Read the model definition and answer for the solid it produces. Units are mm, in the model's axes. Face numbers are marked on the shaded views. A direction names the side the tool comes from. Coordinates: 2 decimals unless noted, no trailing zeros. Write each loop counter-clockwise with the first axis right and the second up, starting at its lowest first coordinate (ties: lowest second). Pieces come first, ordered by that corner, then holes. Notation, with made-up numbers: M 40,47 L 97,47 A8 ccw 97,57 Z; hole C 25,11 d6. An arc over 180 degrees is marked long. Use a Markdown table: item, result. Add a question column.
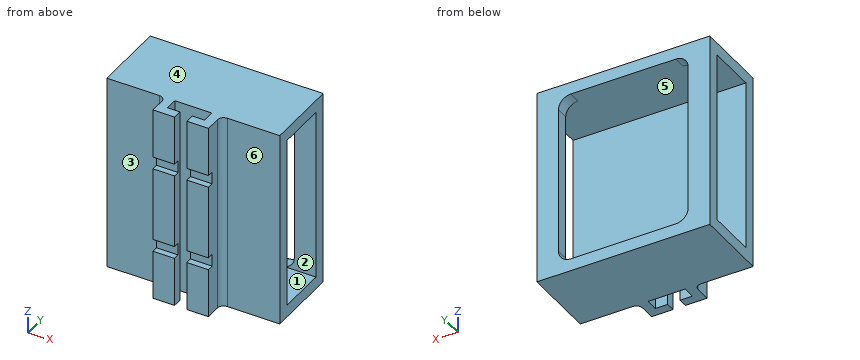
from build123d import *

# Parameters (mm, degrees)
SKETCH_1_W          = 28
SKETCH_1_H          = 12
SKETCH_1_W_2        = 9
SKETCH_1_H_2        = 3.5
EXTRUDE_1_DEPTH     = 32
SKETCH_2_W          = 1
SKETCH_2_H          = 1.5
CUT_EXTRUDE_1_DEPTH = 37.197375595
SKETCH_3_W          = 2
SKETCH_3_H          = 1
CUT_EXTRUDE_2_DEPTH = 39.164119275
FILLET_1_R          = 1
SKETCH_6_W          = 28
SKETCH_6_H          = 8
CUT_EXTRUDE_5_DEPTH = 44.568910934
CUT_EXTRUDE_4_REACH = 40.213
SKETCH_5_W          = 21
SKETCH_5_H          = 28
FILLET_2_R          = 2


with BuildPart() as part:
    # 草图1 → 凸台-拉伸1 (new body)
    with BuildSketch(Plane.XY):
        Rectangle(SKETCH_1_W, SKETCH_1_H)
        with Locations((0, -7.75)):
            Rectangle(SKETCH_1_W_2, SKETCH_1_H_2)
    extrude(amount=EXTRUDE_1_DEPTH)

    # 草图2 → 切除-拉伸1 (cut, through all)
    with BuildSketch(Plane(origin=(0, 0, 0), x_dir=(-1, 0, 0), z_dir=(0, 0, -1))):
        Polygon((0, -6), (-3, -6), (-3, -8), (-1, -8), (0, -8), align=None)
        Polygon((3, -6), (0, -6), (0, -8), (1, -8), (3, -8), align=None)
        with Locations((-0.5, -8.75)):
            Rectangle(SKETCH_2_W, SKETCH_2_H)
        with Locations((0.5, -8.75)):
            Rectangle(SKETCH_2_W, SKETCH_2_H)
    extrude(amount=-CUT_EXTRUDE_1_DEPTH, mode=Mode.SUBTRACT)

    # 草图3 → 切除-拉伸2 (cut, through all)
    with BuildSketch(Plane.ZY.offset(4.5)):
        with Locations((9, -9)):
            Rectangle(SKETCH_3_W, SKETCH_3_H)
        with Locations((23, -9)):
            Rectangle(SKETCH_3_W, SKETCH_3_H)
    extrude(amount=-CUT_EXTRUDE_2_DEPTH, mode=Mode.SUBTRACT)

    # 圆角1
    fillet_1_edges = [part.edges().sort_by_distance(p)[0] for p in [
        (4.5, -6, 16),
        (-4.5, -6, 16),
    ]]
    fillet(fillet_1_edges, radius=FILLET_1_R)

    # 草图6 → 切除-拉伸5 (cut, through all)
    with BuildSketch(Plane(origin=(14, 0, 0), x_dir=(0, 0, -1), z_dir=(1, 0, 0))):
        with Locations((-16, 0)):
            Rectangle(SKETCH_6_W, SKETCH_6_H)
    extrude(amount=-CUT_EXTRUDE_5_DEPTH, mode=Mode.SUBTRACT)

    # 草图5 → 切除-拉伸4 (cut, up to next)
    with BuildSketch(Plane(origin=(0, 6, 0), x_dir=(1, 0, 0), z_dir=(0, 1, 0)), mode=Mode.PRIVATE) as cut_extrude_4_sk1:
        with Locations((0, -16)):
            Rectangle(SKETCH_5_W, SKETCH_5_H)
    cut_extrude_4_tool1 = extrude(cut_extrude_4_sk1.sketch, amount=-CUT_EXTRUDE_4_REACH, mode=Mode.PRIVATE) & part.part
    add(cut_extrude_4_tool1.solids().sort_by_distance((0, 6, 16))[0], mode=Mode.SUBTRACT)

    # 圆角2
    fillet_2_edges = [part.edges().sort_by_distance(p)[0] for p in [
        (10.5, 5, 30),
        (10.5, 5, 2),
        (-10.5, 5, 2),
        (-10.5, 5, 30),
    ]]
    fillet(fillet_2_edges, radius=FILLET_2_R)


solid = part.part
Item 1: Find section B-B on z = 15. Give the vertices of the cut face in (x, y), then the cut area to 3 significant figures.
Item 2: Find section C-C on x = -2.25. Give the vertices of the cut face in (y, z), then the cut area to 3 significant figures.
Item 3: Each of these flat-tipped pins is pushed along its axis until it touches: pin 1 (4 mm diameter, centred on x = 12, z = 8, fed in from -Y); pin 2 (2 mm diameter, centred on y = -7.5, z = 10, fed in from +X); pin 3 (1.5 mm diameter, centred on x = 1, z = 11, fed in from +Y); pin 4 (0.8 mm diameter, centred on x = -3, y = -9, fed in from -Z). Where does it stop, or does it pass through?
Item 4: Consider probe 1 along Z at (x, y) = (9, 3.25); probe 2 along Y at (x, z) = (11, 28); probe 3 along Y at (x, z) = (-10, 14.5). Determine where each line is inside the solid, lowest interval first.
Item 5: Find section A-A on y = 2.75. Give the vertices of the cut face in (x, z), then the cut area to 3 significant figures.
Item 6: Determine the mould class of the marked faces 4, 5 and 6 for opening direction Z: pulls with the +Z half, pulls with the -Z half, needs draft (parallel to the pull), parting line crosses it, or undercut.
Item 7: For the marked faces 1, 2 and 3, determine the directions among +Z, -Z, +X, -X, +Y, -Y from which every point of the face is accessible in a straight line to the end or side of a thin tool.
Item 8: Find section D-D on x = 6.5. Give the vertices of the cut face in (y, z).
Geometry says:
| question | item | result |
|---|---|---|
| 1 | outline | M -14,-6 L -5.5,-6 A1 cw -4.5,-7 L -4.5,-9.5 L -1,-9.5 L -1,-8 L -3,-8 L -3,-6 L 3,-6 L 3,-8 L 1,-8 L 1,-9.5 L 4.5,-9.5 L 4.5,-7 A1 cw 5.5,-6 L 14,-6 L 14,-4 L -14,-4 Z; M -14,4 L -10.5,4 L -10.5,6 L -14,6 Z; M 10.5,4 L 14,4 L 14,6 L 10.5,6 Z |
| 1 | area | 86.9 mm2 |
| 2 | outline | M -9.5,0 L -8,0 L -8,32 L -9.5,32 L -9.5,24 L -8.5,24 L -8.5,22 L -9.5,22 L -9.5,10 L -8.5,10 L -8.5,8 L -9.5,8 Z; M -6,0 L 6,0 L 6,2 L -4,2 L -4,30 L 6,30 L 6,32 L -6,32 Z |
| 2 | area | 148 mm2 |
| 3 | pin 1 | stops at y = -6 |
| 3 | pin 2 | stops at x = 4.63 |
| 3 | pin 3 | stops at y = -4 |
| 3 | pin 4 | stops at z = 0 |
| 4 | probe 1 | z = 0 to 2, 30 to 32 |
| 4 | probe 2 | y = -6 to -4, 4 to 6 |
| 4 | probe 3 | y = -6 to -4 |
| 5 | outline | M -14,0 L 14,0 L 14,2 L -14,2 Z; M -14,30 L 14,30 L 14,32 L -14,32 Z |
| 5 | area | 112 mm2 |
| 6 | face 4 | pulls with the +Z half |
| 6 | face 5 | undercut |
| 6 | face 6 | needs draft |
| 7 | face 1 | none |
| 7 | face 2 | +X, -X |
| 7 | face 3 | +Z, -Z, -X, -Y |
| 8 | outline | M -6,0 L 6,0 L 6,2 L -4,2 L -4,30 L 6,30 L 6,32 L -6,32 Z |
